Design review of the part built by this model. Coordinates are the model's own, in mm. A direction names the side the tool comes from. Round coordinates to 2 decimals unless told otherwise and drop trailing zeros. Order: outer loops, then holes, each group sorted by start corner. A loop starts at its lowest first (then second) coordinate and runs counter-clockwise, first axis right, second up. Notation, with made-up numbers: (29, 77.5) - (51, 77.5) arc R24 ccw to (51, 96.5) - close; hole circle Ø10 at (11.25, 76.5). An arc over 180 degrees is marked (long way). Write item = value, one per line.
Autodesk Fusion 360 part; units mm, degrees
sketch "baseplate" plane through (0, 0, 0) normal (0, 1, 0) x (1, 0, 0)
  line L0 (0, 0) -> (80, 0)
  line L1 (80, 0) -> (80, -40)
  line L2 (80, -40) -> (0, -40)
  line L3 (0, -40) -> (0, 0)
  dimension "d1" = 40
  dimension "d2" = 80
extrude "Extrude1" add sketch "baseplate" along normal blind 10
sketch "outside_pryamid" plane through (0, 0, 0) normal (0, 1, 0) x (1, 0, 0)
  line L0 (5, -35) -> (15, -35)
  line L1 (15, -35) -> (15, -25)
  line L2 (15, -25) -> (5, -25)
  line L3 (5, -25) -> (5, -35)
  line L4 (25, -35) -> (35, -35)
  line L5 (35, -35) -> (35, -25)
  line L6 (35, -25) -> (25, -25)
  line L7 (25, -25) -> (25, -35)
  line L8 (45, -35) -> (55, -35)
  line L9 (55, -35) -> (55, -25)
  line L10 (55, -25) -> (45, -25)
  line L11 (45, -25) -> (45, -35)
  line L12 (65, -35) -> (75, -35)
  line L13 (75, -35) -> (75, -25)
  line L14 (75, -25) -> (65, -25)
  line L15 (65, -25) -> (65, -35)
  line L16 (25, -15) -> (35, -15)
  line L17 (35, -15) -> (35, -5)
  line L18 (35, -5) -> (25, -5)
  line L19 (25, -5) -> (25, -15)
  line L20 (5, -15) -> (15, -15)
  line L21 (15, -15) -> (15, -5)
  line L22 (15, -5) -> (5, -5)
  line L23 (5, -5) -> (5, -15)
  line L24 (45, -15) -> (55, -15)
  line L25 (55, -15) -> (55, -5)
  line L26 (55, -5) -> (45, -5)
  line L27 (45, -5) -> (45, -15)
  line L28 (65, -15) -> (75, -15)
  line L29 (75, -15) -> (75, -5)
  line L30 (75, -5) -> (65, -5)
  line L31 (65, -5) -> (65, -15)
  dimension "d5" = 10
  dimension "d6" = 10
ref_plane "WorkPlane1" through (0, 5, 0) normal (0, 1, 0) x (0, 0, 1)
sketch "inside_pryamid" plane through (0, 5, 0) normal (0, 1, 0) x (1, 0, 0)
  line L0 (7.5, -10) -> (7.5, -12.5)
  line L1 (7.5, -12.5) -> (12.5, -12.5)
  line L2 (12.5, -12.5) -> (12.5, -7.5)
  line L3 (12.5, -7.5) -> (7.5, -7.5)
  line L4 (7.5, -7.5) -> (7.5, -10)
  line L5 (32.5, -7.5) -> (27.5, -7.5)
  line L6 (27.5, -10) -> (27.5, -12.5)
  line L7 (32.5, -12.5) -> (32.5, -7.5)
  line L8 (27.5, -7.5) -> (27.5, -10)
  line L9 (27.5, -12.5) -> (32.5, -12.5)
  line L10 (47.5, -7.5) -> (47.5, -10)
  line L11 (47.5, -12.5) -> (52.5, -12.5)
  line L12 (52.5, -7.5) -> (47.5, -7.5)
  line L13 (47.5, -10) -> (47.5, -12.5)
  line L14 (52.5, -12.5) -> (52.5, -7.5)
  line L15 (67.5, -10) -> (67.5, -12.5)
  line L16 (67.5, -12.5) -> (72.5, -12.5)
  line L17 (67.5, -7.5) -> (67.5, -10)
  line L18 (72.5, -12.5) -> (72.5, -7.5)
  line L19 (72.5, -7.5) -> (67.5, -7.5)
  line L20 (67.5, -10) -> (67.5, -12.5)
  line L21 (7.5, -7.5) -> (7.5, -10)
  line L22 (12.5, -7.5) -> (7.5, -7.5)
  line L23 (7.5, -10) -> (7.5, -12.5)
  line L24 (67.5, -12.5) -> (72.5, -12.5)
  line L25 (27.5, -10) -> (27.5, -12.5)
  line L26 (27.5, -12.5) -> (32.5, -12.5)
  line L27 (7.5, -12.5) -> (12.5, -12.5)
  line L28 (32.5, -12.5) -> (32.5, -7.5)
  line L29 (72.5, -12.5) -> (72.5, -7.5)
  line L30 (47.5, -7.5) -> (47.5, -10)
  line L31 (52.5, -12.5) -> (52.5, -7.5)
  line L32 (72.5, -7.5) -> (67.5, -7.5)
  line L33 (47.5, -10) -> (47.5, -12.5)
  line L34 (52.5, -7.5) -> (47.5, -7.5)
  line L35 (67.5, -7.5) -> (67.5, -10)
  line L36 (47.5, -12.5) -> (52.5, -12.5)
  line L37 (32.5, -7.5) -> (27.5, -7.5)
  line L38 (27.5, -7.5) -> (27.5, -10)
  line L39 (12.5, -12.5) -> (12.5, -7.5)
  line L40 (72.5, -32.5) -> (72.5, -27.5)
  line L41 (12.5, -32.5) -> (12.5, -27.5)
  line L42 (72.5, -27.5) -> (67.5, -27.5)
  line L43 (7.5, -30) -> (7.5, -32.5)
  line L44 (67.5, -30) -> (67.5, -32.5)
  line L45 (72.5, -27.5) -> (67.5, -27.5)
  line L46 (67.5, -27.5) -> (67.5, -30)
  line L47 (47.5, -30) -> (47.5, -32.5)
  line L48 (12.5, -27.5) -> (7.5, -27.5)
  line L49 (67.5, -27.5) -> (67.5, -30)
  line L50 (67.5, -30) -> (67.5, -32.5)
  line L51 (7.5, -32.5) -> (12.5, -32.5)
  line L52 (67.5, -32.5) -> (72.5, -32.5)
  line L53 (72.5, -32.5) -> (72.5, -27.5)
  line L54 (7.5, -30) -> (7.5, -32.5)
  line L55 (47.5, -32.5) -> (52.5, -32.5)
  line L56 (47.5, -32.5) -> (52.5, -32.5)
  line L57 (67.5, -32.5) -> (72.5, -32.5)
  line L58 (52.5, -32.5) -> (52.5, -27.5)
  line L59 (7.5, -32.5) -> (12.5, -32.5)
  line L60 (52.5, -27.5) -> (47.5, -27.5)
  line L61 (52.5, -27.5) -> (47.5, -27.5)
  line L62 (47.5, -30) -> (47.5, -32.5)
  line L63 (7.5, -27.5) -> (7.5, -30)
  line L64 (27.5, -30) -> (27.5, -32.5)
  line L65 (32.5, -27.5) -> (27.5, -27.5)
  line L66 (27.5, -32.5) -> (32.5, -32.5)
  line L67 (52.5, -32.5) -> (52.5, -27.5)
  line L68 (27.5, -27.5) -> (27.5, -30)
  line L69 (32.5, -32.5) -> (32.5, -27.5)
  line L70 (27.5, -32.5) -> (32.5, -32.5)
  line L71 (27.5, -30) -> (27.5, -32.5)
  line L72 (12.5, -27.5) -> (7.5, -27.5)
  line L73 (7.5, -27.5) -> (7.5, -30)
  line L74 (47.5, -27.5) -> (47.5, -30)
  line L75 (12.5, -32.5) -> (12.5, -27.5)
  line L76 (47.5, -27.5) -> (47.5, -30)
  line L77 (32.5, -32.5) -> (32.5, -27.5)
  line L78 (32.5, -27.5) -> (27.5, -27.5)
  line L79 (27.5, -27.5) -> (27.5, -30)
loft "Loft1" cut profiles "outside_pryamid", "inside_pryamid" section 1 contours L0 L1 L2 L3 section 2 contours L41 L43 L48 L51 L54 L59 L63 L72 L73 L75
loft "Loft2" cut profiles "outside_pryamid", "inside_pryamid" section 1 contours L4 L5 L6 L7 section 2 contours L64 L65 L66 L68 L69 L70 L71 L77 L78 L79
loft "Loft3" cut profiles "outside_pryamid", "inside_pryamid" section 1 contours L8 L9 L10 L11 section 2 contours L47 L55 L56 L58 L60 L61 L62 L67 L74 L76
loft "Loft4" cut profiles "inside_pryamid", "outside_pryamid" section 1 contours L40 L42 L44 L45 L46 L49 L50 L52 L53 L57 section 2 contours L12 L13 L14 L15
loft "Loft5" cut profiles "inside_pryamid", "outside_pryamid" section 1 contours L0 L1 L2 L3 L4 L21 L22 L23 L27 L39 section 2 contours L20 L21 L22 L23
loft "Loft6" cut profiles "inside_pryamid", "outside_pryamid" section 1 contours L5 L6 L7 L8 L9 L25 L26 L28 L37 L38 section 2 contours L16 L17 L18 L19
loft "Loft7" cut profiles "inside_pryamid", "outside_pryamid" section 1 contours L10 L11 L12 L13 L14 L30 L31 L33 L34 L36 section 2 contours L24 L25 L26 L27
loft "Loft8" cut profiles "inside_pryamid", "outside_pryamid" section 1 contours L15 L16 L17 L18 L19 L20 L24 L29 L32 L35 section 2 contours L28 L29 L30 L31
sketch "sidewall" plane through (0, 0, 0) normal (0, 1, 0) x (1, 0, 0)
  line L0 (0, 0) -> (-8, 0)
  line L1 (-8, 0) -> (-8, -40)
  line L2 (-8, -40) -> (0, -40)
  line L3 (0, -40) -> (0, 0)
  dimension "d12" = 8
extrude "Extrude2" add sketch "sidewall" along normal blind -40 and the other way blind -10
sketch "sidemount" plane through (0, 0, 0) normal (0, 1, 0) x (1, 0, 0)
  line L0 (80, 0) -> (88, 0)
  line L1 (88, 0) -> (88, -40)
  line L2 (88, -40) -> (80, -40)
  line L3 (80, -40) -> (80, 0)
extrude "Extrude3" add sketch "sidemount" along normal blind 10
sketch "Sketch6" plane through (0, 0, 0) normal (0, 1, 0) x (1, 0, 0)
  circle A0 centre (-4, -34) radius 2
  circle A1 centre (-4, -6) radius 2
  circle A2 centre (-4, -34) radius 3.4
  circle A3 centre (-4, -6) radius 3.4
  line L0 (88, 0) -> (84, 0)
  line L1 (84, 0) -> (84, -6)
  line L2 (84, -6) -> (88, -6)
  line L3 (88, -6) -> (88, 0)
  circle A4 centre (84, -34) radius 2
  circle A5 centre (84, -6) radius 2
  dimension "d19" = 4
  dimension "d20" = 4
  dimension "d21" = 6.8
  dimension "d22" = 6.8
  dimension "d25" = 4
  dimension "d26" = 6
  dimension "d27" = 4
  dimension "d28" = 4
extrude "Extrude4" cut sketch "Sketch6" against normal blind 50 contours A0 | A1
extrude "Extrude5" cut sketch "Sketch6" along normal blind 40 contours L1 L2 A5 | L1 L2 A5 | A4
extrude "Extrude6" cut sketch "Sketch6" along normal through all and the other way blind 44 contours A0 | A1
extrude "Extrude7" cut sketch "Sketch6" along normal blind 10 and the other way blind -4 contours A2 | A3
1) We need section A-A on x = -4. Write out the cut boundary in (y, z), and give its area (3 significant figures).
Findings:
outline = (-40, 0) - (10, 0) - (10, 2.6) - (4, 2.6) - (4, 4) - (-40, 4) - close; (-40, 8) - (4, 8) - (4, 9.4) - (10, 9.4) - (10, 30.6) - (4, 30.6) - (4, 32) - (-40, 32) - close; (-40, 36) - (4, 36) - (4, 37.4) - (10, 37.4) - (10, 40) - (-40, 40) - close
area = 1,570 mm^2
2) We need section D-D on z = 34. Give the number of separate pieces and of enclosed holes in the cut face, and give its area (3 significant figures).
Findings:
separate_pieces = 3
enclosed_holes = 0
area = 951 mm^2
3) We need section B-B on y = -15.5. Write out the cut boundary in (x, z).
Findings:
outline = (-8, 0) - (0, 0) - (0, 40) - (-8, 40) - close; hole circle Ø4 at (-4, 6); hole circle Ø4 at (-4, 34)
4) We need section C-C on x = 84. Write out the cut boundary in (y, z), and give its area (3 significant figures).
Findings:
outline = (0, 0) - (10, 0) - (10, 4) - (0, 4) - close; (0, 8) - (10, 8) - (10, 32) - (0, 32) - close; (0, 36) - (10, 36) - (10, 40) - (0, 40) - close
area = 320 mm^2
5) The part is to be moulded in two halves that separate along Z. For faces 1 (the flat face through (26, 2, 30)), 2 (the flat face through (43, 0, 20)), 3 (the flat face through (29, 2, 0)), 4 (the flat face through (30, 2, 40)), say which applies: released by +Z, released by -Z, zero draft, split by the parting line, or undercut.
Findings:
face_1 = undercut
face_2 = zero draft
face_3 = released by -Z
face_4 = released by +Z
6) For faces 5 (the flat face through (-4, 4, 8.2)), 6 (the flat face through (26, 2, 10)), 7 (the flat face through (0, -20, 20)), 8 (the cylindrical face through (-4, -18, 36)), list the 3-axis set-ups (+Z, -Z, +X, -X, +Y, -Y) from which the entire face can be reached by the end or side of a thin tool; tool diameter is ignored.
Findings:
face_5 = +Y
face_6 = -Y
face_7 = +Z, -Z, +X, -Y
face_8 = +Y, -Y
7) Clearance check with flat-ended pins moving along their axes: pin 1 Ø20 at (y, z) = (-27.5, 11.5) entering from +X; pin 2 Ø5.5 at (x, z) = (9.5, 9) entering from -Y; pin 3 Ø12 at (x, z) = (62, 7) entering from -Y. State where each tip first meets the part, or that it passes through.
Findings:
pin_1 = 0
pin_2 = 2.5
pin_3 = 0
8) To check wall thickness, follow L1, parallel to X at y = 6, z = 6; L2, parallel to Z at x = 84, y = 3.75; L3, parallel to X at y = 3, z = 6. State the ranges of each line that lie inside material, in increasing order. Write a range as from..to.
Findings:
L1 = -8..-7.4, -0.6..82, 86..88
L2 = 0..4, 8..32, 36..40
L3 = -8..-6, -2..82, 86..88
